from build123d import *

# Parameters (mm, degrees)
F0_W     = 83.34375
F0_H     = 7.9375
F0_W_2   = 80.9625
F0_W_3   = 7.9375
F1_DEPTH = 165.1
F0_H_2   = 73.025
F2_DEPTH = 1.5875
F3_DEPTH = 107.95


with BuildPart() as f1:
    # F0 (on Top) → F1 (new body)
    with BuildSketch(Plane.XY):
        with Locations((-90.090625, 84.93125)):
            Rectangle(F0_W, F0_H)
        with Locations((0, 84.93125)):
            Rectangle(F0_W_2, F0_H)
        Polygon((-48.41875, 88.9), (-48.41875, 80.9625), (-40.48125, 80.9625), (-40.48125, 88.9), (-44.45, 88.9), align=None)
        with Locations((-135.73125, 84.93125)):
            Rectangle(F0_W_3, F0_H)
        Polygon((40.48125, 88.9), (40.48125, 80.9625), (48.41875, 80.9625), (48.41875, 88.9), (44.45, 88.9), align=None)
        with Locations((90.090625, 84.93125)):
            Rectangle(F0_W, F0_H)
        with Locations((135.73125, 84.93125)):
            Rectangle(F0_W_3, F0_H)
    extrude(amount=F1_DEPTH)


with BuildPart() as f2:
    # F0 (on Top) → F2 (new body)
    with BuildSketch(Plane.XY):
        with Locations((-90.090625, 44.45)):
            Rectangle(F0_W, F0_H_2)
    extrude(amount=F2_DEPTH)


with BuildPart() as f2b:
    # F0 (on Top) → F2, piece 2 (new body)
    with BuildSketch(Plane.XY):
        with Locations((0, 44.45)):
            Rectangle(F0_W_2, F0_H_2)
    extrude(amount=F2_DEPTH)


with BuildPart() as f2c:
    # F0 (on Top) → F2, piece 3 (new body)
    with BuildSketch(Plane.XY):
        with Locations((90.090625, 44.45)):
            Rectangle(F0_W, F0_H_2)
    extrude(amount=F2_DEPTH)


with BuildPart() as f3:
    # F0 (on Top) → F3 (new body)
    with BuildSketch(Plane.XY):
        Polygon((-48.41875, 88.9), (-48.41875, 80.9625), (-40.48125, 80.9625), (-40.48125, 88.9), (-44.45, 88.9), align=None)
        with Locations((-44.45, 44.45)):
            Rectangle(F0_W_3, F0_H_2)
        Polygon((-48.41875, 7.9375), (-48.41875, 0), (-44.45, 0), (-40.48125, 0), (-40.48125, 7.9375), align=None)
        Polygon((40.48125, 7.9375), (40.48125, 0), (44.45, 0), (48.41875, 0), (48.41875, 7.9375), align=None)
        with Locations((44.45, 44.45)):
            Rectangle(F0_W_3, F0_H_2)
        Polygon((40.48125, 88.9), (40.48125, 80.9625), (48.41875, 80.9625), (48.41875, 88.9), (44.45, 88.9), align=None)
        with Locations((135.73125, 44.45)):
            Rectangle(F0_W_3, F0_H_2)
        with Locations((-135.73125, 44.45)):
            Rectangle(F0_W_3, F0_H_2)
        with Locations((-90.090625, 3.96875)):
            Rectangle(F0_W, F0_H)
        Polygon((-139.7, 5.3547988646), (-139.7, 0), (-131.7625, 0), (-131.7625, 7.9375), (-139.7, 7.9375), align=None)
        with Locations((-135.73125, 84.93125)):
            Rectangle(F0_W_3, F0_H)
        with Locations((-90.090625, 84.93125)):
            Rectangle(F0_W, F0_H)
        with Locations((0, 84.93125)):
            Rectangle(F0_W_2, F0_H)
        with Locations((0, 3.96875)):
            Rectangle(F0_W_2, F0_H)
        with Locations((90.090625, 3.96875)):
            Rectangle(F0_W, F0_H)
        with Locations((135.73125, 3.96875)):
            Rectangle(F0_W_3, F0_H)
        with Locations((135.73125, 84.93125)):
            Rectangle(F0_W_3, F0_H)
        with Locations((90.090625, 84.93125)):
            Rectangle(F0_W, F0_H)
    extrude(amount=F3_DEPTH)


with BuildPart() as f1_1:
    add(f1.part)

    # F4: union F2c, F2, F3, F2b
    add(f2c.part)
    add(f2.part)
    add(f3.part)
    add(f2b.part)

    # F6: F1 across plane


with BuildPart() as f1_2:
    add(f1_1.part)
    add(f1_1.part.mirror(Plane.XZ.offset(-84.93125)))


solid = f1_2.part
Here's how the part is built. I have some questions about the finished solid (model axes, mm). A direction names the side the tool comes from. Coordinates: 2 decimals unless noted, no trailing zeros. Write each loop counter-clockwise with the first axis right and the second up, starting at its lowest first coordinate (ties: lowest second). Pieces come first, ordered by that corner, then holes. Notation, with made-up numbers: (-9, 23) - (39, 23) arc R17 ccw to (39, 36) - close; hole circle Ø2 at (36.25, 5.25). An arc over 180 degrees is marked (long way). Use one line per item in the form item = value.
1) Suppose I cut it at B-B, the plane y = 155. Write out the boundary of the cut face in (x, z).
Solved:
outline = (-139.7, 0) - (139.7, 0) - (139.7, 107.95) - (131.76, 107.95) - (131.76, 1.59) - (48.42, 1.59) - (48.42, 107.95) - (40.48, 107.95) - (40.48, 1.59) - (-40.48, 1.59) - (-40.48, 107.95) - (-48.42, 107.95) - (-48.42, 1.59) - (-131.76, 1.59) - (-131.76, 107.95) - (-139.7, 107.95) - close
2) I'm going to push flat-ended pins straight in: P1, Ø22, axis at x = 90, y = 116.5, coming from the +Z side; P2, Ø1, axis at x = -23.5, z = 119, coming from the -Y side; P3, Ø6, axis at x = 2, z = 125.5, coming from the +Y side. Where does each tip first touch, or does it pass through?
Solved:
P1 = 1.59
P2 = 80.96
P3 = 88.9
3) Thinking about a two-plate mould opening in X: for faces 3 (the flat face through (90, 161.925, 54)), 4 (the flat face through (-1, 165, 107.95)), which applies, released by +X, released by -X, zero draft, split by the parting line, or undercut?
Solved:
face_3 = undercut
face_4 = zero draft
4) I need wall thicknesses on line 1 (X direction, y = 150, z = 67.5); line 2 (Y direction, x = -112.5, z = 76) (1 decimal); line 3 (Z direction, x = -30.5, y = 62). Which ranges of each line are inside material? Lowest first, please.
Solved:
line_1 = -139.7 to -131.76, -48.42 to -40.48, 40.48 to 48.42, 131.76 to 139.7
line_2 = 0 to 7.9, 81 to 88.9, 161.9 to 169.9
line_3 = 0 to 1.59
5) Suppose I cut it at A-A, the plane z = 81. Write out the boundary of the cut face in (x, y) (1 decimal).
Solved:
outline = (-139.7, 0) - (139.7, 0) - (139.7, 169.9) - (-139.7, 169.9) - close; hole (-131.8, 7.9) - (-48.4, 7.9) - (-48.4, 81) - (-131.8, 81) - close; hole (-131.8, 88.9) - (-48.4, 88.9) - (-48.4, 161.9) - (-131.8, 161.9) - close; hole (-40.5, 7.9) - (40.5, 7.9) - (40.5, 81) - (-40.5, 81) - close; hole (-40.5, 88.9) - (40.5, 88.9) - (40.5, 161.9) - (-40.5, 161.9) - close; hole (48.4, 7.9) - (131.8, 7.9) - (131.8, 81) - (48.4, 81) - close; hole (48.4, 88.9) - (131.8, 88.9) - (131.8, 161.9) - (48.4, 161.9) - close
6) On a 3-axis mill with a long thin cutter (end or side, diameter ignored), from which of +Z, -Z, +X, -X, +Y, -Y can I reach the whole of each face in a straight line? I mean faces 1 (the flat face through (-1, 125, 1.588)), 2 (the flat face through (-2, 169.862, 53)). Say none if no direction works.
Solved:
face_1 = +Z
face_2 = +Z, -Z, +X, -X, +Y
